Autodesk Inventor part; units mm, degrees
ref_plane "YZ Plane" through (0, 0, 0) normal (1, 0, 0) x (0, 1, 0)
ref_plane "XZ Plane" through (0, 0, 0) normal (0, 1, 0) x (-1, 0, 0)
ref_plane "XY Plane" through (0, 0, 0) normal (0, 0, 1) x (1, 0, 0)
sketch "スケッチ1" plane through (0, 0, 0) normal (0, 0, 1) x (1, 0, 0)
  circle A0 centre (0, 0) radius 3
  circle A1 centre (0, 0) radius 1.5
  dimension "d0" = 6
  dimension "d1" = 3
extrude "押し出し1" add sketch "スケッチ1" along normal blind 40
fillet "フィレット1" radius 0.3 2 edges at (-3, 0, 40) (-3, 0, 0)
thread "ねじ1"
extrude "押し出し2" add sketch "スケッチ1" along normal blind 29 contours A1
extrude "押し出し3" cut sketch "スケッチ1" along normal blind 6 contours A1
thread "ねじ2"
properties part number "スペーサーM3L40アルミ" material "アルミニウム 2014-T4"
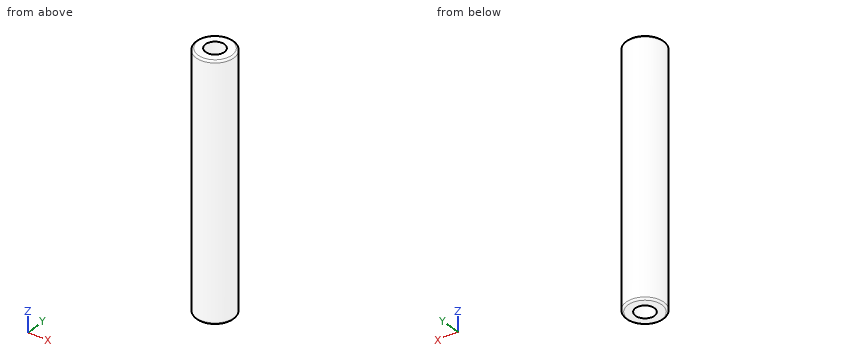
Part model, mm, in its own coordinate system. Round coordinates to 2 decimals unless told otherwise and drop trailing zeros. Order: outer loops, then holes, each group sorted by start corner. A loop starts at its lowest first (then second) coordinate and runs counter-clockwise, first axis right, second up. Notation, with made-up numbers: M 42.5,-29 L 94.5,-29 A16 cw 94.5,-6 Z; hole C 15,-17.75 d4. An arc over 180 degrees is marked long. Put each result on its own line as item: value. Start each with the question number.
1. Drill centre lines: probe 1 along Y at (x, z) = (0, 4.2); probe 2 along X at (y, z) = (-1, 2.5); probe 3 along X at (y, z) = (0.25, 5). Where is each one in solid material? Low to high. Write a range as [from, to].
2. Drop flat-ended pins along their axis: pin 1 (2.5 mm diameter, centred on x = 0, y = 0, fed in from -Z); pin 2 (2 mm diameter, centred on x = 1.5, z = 4.5, fed in from +Y). Give the stop position or say it passes through.
3. Slice it at A-A on x = 0. List the corners of the cut face in (y, z), then the cut area to 3 significant figures.
4. Slice it at C-C on z = 32.5. List the corners of the cut face in (x, y).
5. Slice it at D-D on z = 14. List the corners of the cut face in (x, y), then the cut area to 3 significant figures.
Findings:
1. probe 1: [-3, -1.5], [1.5, 3]
1. probe 2: [-2.83, -1.12], [1.12, 2.83]
1. probe 3: [-2.99, -1.48], [1.48, 2.99]
2. pin 1: z = 6
2. pin 2: y = 2.96
3. outline: M -3,0.3 A0.3 ccw -2.7,0 L -1.5,0 L -1.5,6 L 1.5,6 L 1.5,0 L 2.7,0 A0.3 ccw 3,0.3 L 3,39.7 A0.3 ccw 2.7,40 L 1.5,40 L 1.5,29 L -1.5,29 L -1.5,40 L -2.7,40 A0.3 ccw -3,39.7 Z
3. area: 189 mm2
4. outline: C 0,0 d6; hole C 0,0 d3
5. outline: C 0,0 d6
5. area: 28.3 mm2
